Design review of the part built by this model. Coordinates are the model's own, in mm. A direction names the side the tool comes from. Give positions to 0.01 mm unless a question says otherwise; leave off trailing zeros. Write each loop counter-clockwise with the first axis right and the second up, starting at its lowest first coordinate (ties: lowest second). Pieces come first, ordered by that corner, then holes. Notation, with made-up numbers: M 16.5,-39.75 L 49.5,-39.75 A17 cw 49.5,-32.75 Z; hole C -3.5,18.25 d1. An arc over 180 degrees is marked long. Answer in a Markdown table with one row per item.
```python
from build123d import *

# Parameters (mm, degrees)
EXTRUDE_1_DEPTH = 6


with BuildPart() as part:
    # 草图1 → 凸台-拉伸1 (new body)
    with BuildSketch(Plane.XY):
        with BuildLine():
            Line((0, 5), (23, 5))
            ThreePointArc((23, 5), (28, 0), (23, -5))
            Line((23, -5), (0, -5))
            ThreePointArc((0, -5), (-5, 0), (0, 5))
        make_face()
    extrude(amount=EXTRUDE_1_DEPTH)

    # 草图2 → 切除-旋转1 (revolve, cut)
    with BuildSketch(Plane(origin=(0, 0, 0), x_dir=(1, 0, 0), z_dir=(0, 1, 0))):
        Polygon((0, -6), (-3.75, -6), (-3.75, -2.5), (-2.75, -2.5), (-2.75, 0), (0, 0), align=None)
    revolve(axis=Axis((0, 0, 0), (0, 0, 1)), mode=Mode.SUBTRACT)

    # 草图3 → 切除-旋转2 (revolve, cut)
    with BuildSketch(Plane(origin=(0, 0, 0), x_dir=(1, 0, 0), z_dir=(0, 1, 0))):
        Polygon((23, -6), (19.25, -6), (19.25, -2.5), (20.25, -2.5), (20.25, 0), (23, 0), align=None)
    revolve(axis=Axis((23, 0, 0), (0, 0, 1)), mode=Mode.SUBTRACT)


solid = part.part
```
1) Add section A-A (y = 0). Write out the cut boundary in (x, z).
Geometry says:
| item | result |
|---|---|
| outline | M -5,0 L -2.75,0 L -2.75,2.5 L -3.75,2.5 L -3.75,6 L -5,6 Z; M 2.75,0 L 20.25,0 L 20.25,2.5 L 19.25,2.5 L 19.25,6 L 3.75,6 L 3.75,2.5 L 2.75,2.5 Z; M 25.75,0 L 28,0 L 28,6 L 26.75,6 L 26.75,2.5 L 25.75,2.5 Z |
2) For faces 1 (the face through (1, -3, 2.5)), 2 (the face through (-5, 0, 3)), list the 3-axis set-ups (+Z, -Z, +X, -X, +Y, -Y) from which the entire face can be reached by the end or side of a thin tool; tool diameter is ignored.
Geometry says:
| item | result |
|---|---|
| face 1 | +Z |
| face 2 | +Z, -Z, -X |
3) Add section D-D (x = 21). Write out the cut boundary in (y, z), and give its area (3 significant figures).
Geometry says:
| item | result |
|---|---|
| outline | M -5,0 L -1.89,0 L -1.89,2.5 L -3.17,2.5 L -3.17,6 L -5,6 Z; M 1.89,0 L 5,0 L 5,6 L 3.17,6 L 3.17,2.5 L 1.89,2.5 Z |
| area | 28.4 mm^2 |
4) Insertion check: P1, Ø3, axis at y = 3, z = 1.5, coming from the +X side; P2, Ø2, axis at x = 0.5, y = 1, coming from the +Z side. Each pin has a flat end and moves straight along its axis. Give the tip position at first contact, or say it passes through.
Geometry says:
| item | result |
|---|---|
| P1 | x = 27.77 |
| P2 | through |
5) To check wall thickness, follow probe 1 along X at (y, z) = (0, 1.3); probe 2 along X at (y, z) = (0, 4.5); probe 3 along Y at (x, z) = (0, 4.85). State the ranges of each line that lie inside material, in increasing order. Write a range as [from, to].
Geometry says:
| item | result |
|---|---|
| probe 1 | [-5, -2.75], [2.75, 20.25], [25.75, 28] |
| probe 2 | [-5, -3.75], [3.75, 19.25], [26.75, 28] |
| probe 3 | [-5, -3.75], [3.75, 5] |
6) Add section C-C (x = -1). Write out the cut boundary in (y, z), and give its area (3 significant figures).
Geometry says:
| item | result |
|---|---|
| outline | M -4.9,0 L -2.56,0 L -2.56,2.5 L -3.61,2.5 L -3.61,6 L -4.9,6 Z; M 2.56,0 L 4.9,0 L 4.9,6 L 3.61,6 L 3.61,2.5 L 2.56,2.5 Z |
| area | 20.7 mm^2 |
7) Add section B-B (z = 0.9). Write out the cut boundary in (x, y).
Geometry says:
| item | result |
|---|---|
| outline | M 0,-5 L 23,-5 A5 ccw 23,5 L 0,5 A5 ccw Z; hole C 0,0 d5.5; hole C 23,0 d5.5 |
